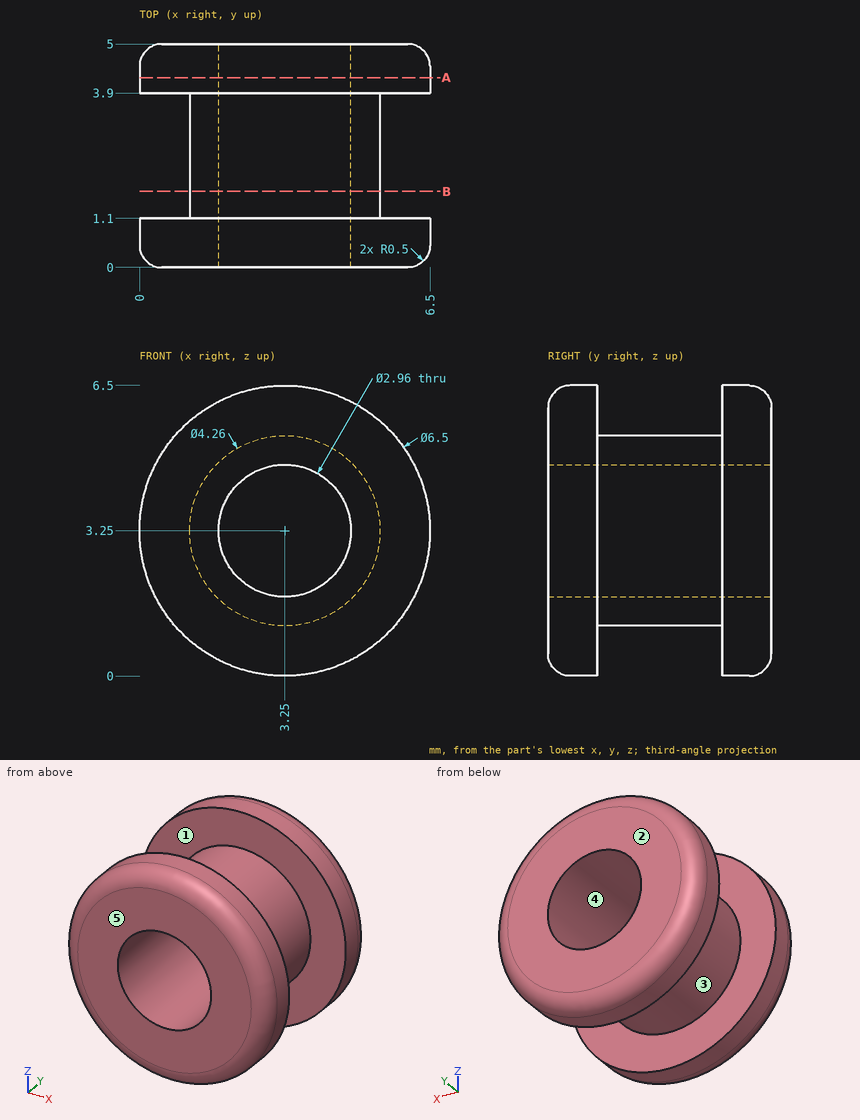
Input: dimensioned drawing with shaded views. Units: mm. Origin: part minimum x, y, z. A direction names the side the tool comes from. Give positions to 0.01 mm unless a question says otherwise; leave off trailing zeros. Write each loop counter-clockwise with the first axis right and the second up, starting at its lowest first coordinate (ties: lowest second). Pieces come first, ordered by that corner, then holes.
1. Pin query (flat end, axial travel): P1, Ø1, axis at x = 1.5, y = 3, coming from the +Z side; P2, Ø1, axis at y = 3, z = 3.5, coming from the +X side; P3, Ø1, axis at y = 4.5, z = 0.5, coming from the +X side. Return the tip coordinate at first contact, or that it passes through.
2. Line query: probe 1 along Y at (x, z) = (0.75, 4.5); probe 2 along Z at (x, y) = (3.25, 1.6); probe 3 along X at (y, z) = (4.15, 2.75). Output: solid intervals per line, ascending.
3. Section query B-B, the plane y = 1.7. Return loops of the section in (x, z), then the cut area to 3 significant figures.
4. Section query A-A, the plane y = 4.25. Return loops of the section in (x, z), then the cut area to 3 significant figures.
5. Draft query along Y for the marked faces 3, 4 and 5. Return one class per face: released by +Y, released by -Y, zero draft, split by the parting line, or undercut.
6. Reachability of the marked faces 1 and 2 from +Z, -Z, +X, -X, +Y, -Y: full face, straight path, thin tool, end or side. Return the list, or none.
Computed:
1. P1: stops at z = 4.97
1. P2: stops at x = 5.38
1. P3: stops at x = 5.6
2. probe 1: y = 0 to 1.1, 3.9 to 5
2. probe 2: z = 1.12 to 1.77, 4.73 to 5.38
2. probe 3: x = 0.04 to 1.86, 4.64 to 6.46
3. outline: circle Ø4.26 at (3.25, 3.25); hole circle Ø2.96 at (3.25, 3.25)
3. area: 7.37 mm2
4. outline: circle Ø6.5 at (3.25, 3.25); hole circle Ø2.96 at (3.25, 3.25)
4. area: 26.3 mm2
5. face 3: undercut
5. face 4: zero draft
5. face 5: released by -Y
6. face 1: none
6. face 2: +Z, -Z, +X, -X, +Y
